Here's how the part is built. I have some questions about the finished solid (model axes, mm). Round coordinates to 2 decimals unless told otherwise and drop trailing zeros. Loops run counter-clockwise (first coordinate to the right, second up) from the corner with the lowest first, then second, coordinate; pieces in that order, holes last. Notation, with made-up numbers: M -1.75,70 L 53.25,70 A10 cw 53.25,87 Z; hole C -5.5,8 d6. An arc over 180 degrees is marked long. Answer as a JSON object with one key per item and string values.
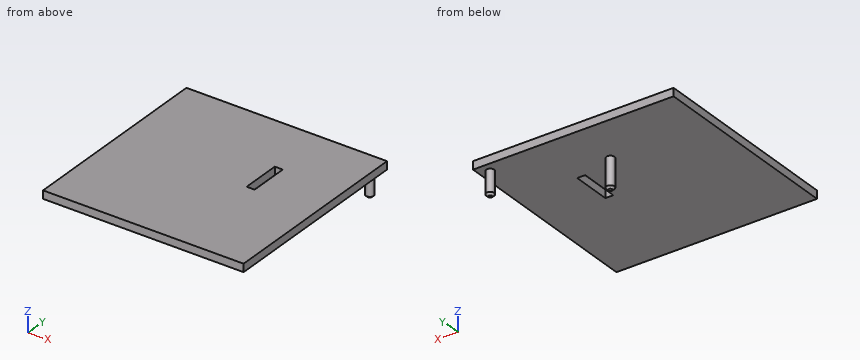
from build123d import *

# Parameters (mm, degrees)
F0_W          = 63.5
F0_H          = 63.5
F0_R          = 1.27
F0_W_2        = 2.54
F0_H_2        = 12.446
F1_DEPTH      = 2.54
F2_R          = 1.27
F3_DEPTH      = 2.54
F3_DEPTH_BACK = 7.62
F4_DEPTH      = 9.525
F5_SIZE       = 0.6477


with BuildPart() as f1:
    # F0 (on Top) → F1 (new body)
    with BuildSketch(Plane.XY):
        with Locations((31.75, 31.75)):
            Rectangle(F0_W, F0_H)
        with Locations((31.353125, 47.625)):
            Circle(F0_R, mode=Mode.SUBTRACT)
        with Locations((42.8625, 38.227)):
            Rectangle(F0_W_2, F0_H_2, mode=Mode.SUBTRACT)
        with Locations((60.325, 60.325)):
            Circle(F0_R, mode=Mode.SUBTRACT)
    extrude(amount=F1_DEPTH)

    # F2 (on Top) → F3 (join, two sides)
    with BuildSketch(Plane.XY) as f3_sk:
        with Locations((31.353125, 47.625)):
            Circle(F2_R)
        with Locations((60.325, 60.325)):
            Circle(F2_R)
    extrude(amount=F3_DEPTH)
    extrude(f3_sk.sketch, amount=-F3_DEPTH_BACK)

    # F2 (on Top) → F4 (join)
    with BuildSketch(Plane.XY):
        with Locations((31.353125, 47.625)):
            Circle(F2_R)
    extrude(amount=-F4_DEPTH)

    # F5
    f5_edges = [f1.edges().sort_by_distance(p)[0] for p in [
        (59.055, 60.325, -7.62),
        (30.083125, 47.625, -9.525),
    ]]
    chamfer(f5_edges, length=F5_SIZE)


solid = f1.part
Item 1: I'm going to push flat-ended pins straight in: pin 1 Ø1.4 at (x, y) = (60.5, 60.5) entering from -Z; pin 2 Ø10 at (x, y) = (41, 33.5) entering from -Z. Where does each tip first touch, or does it pass through?
Resolved:
{"pin 1": "z = -7.62", "pin 2": "z = 0"}
Item 2: I want a section at B-B, the plane x = 36.5. Please give me the cut outline in (y, z), then the cut area to 3 significant figures.
Resolved:
{"outline": "M 0,0 L 63.5,0 L 63.5,2.54 L 0,2.54 Z", "area": "161 mm²"}
Item 3: I want a section at A-A, the plane y = 42. Please give me the cut outline in (x, z).
Resolved:
{"outline": "M 0,0 L 41.59,0 L 41.59,2.54 L 0,2.54 Z; M 44.13,0 L 63.5,0 L 63.5,2.54 L 44.13,2.54 Z"}
Item 4: Please list where this line runs through material, in increasing order: probe 1 along Z at (x, y) = (56.5, 45). Write a range as from..to.
Resolved:
{"probe 1": "0..2.54"}
Item 5: I want a section at D-D, the plane z = -3.5. Please give me the cut outline in (x, y) (3 decimals), then the cut area to 3 significant figures.
Resolved:
{"outline": "C 31.353,47.625 d2.54; C 60.325,60.325 d2.54", "area": "10.1 mm²"}
